Read the model definition and answer for the solid it produces. Units are mm, in the model's axes. A direction names the side the tool comes from. Give positions to 0.01 mm unless a question says otherwise; leave off trailing zeros. Loops run counter-clockwise (first coordinate to the right, second up) from the corner with the lowest first, then second, coordinate; pieces in that order, holes last. Notation, with made-up numbers: (24, 27.5) -> (72, 27.5) arc R24 ccw to (72, 49.5) -> close; hole circle Ø5 at (27, -22.5). An arc over 180 degrees is marked (long way). Write each question's results on one line, items separated by ' | '. Start each with the question number.
Item 1: Section C-C on y = 861 is taken. Write down the section's boundary in (x, z).
Item 2: Section A-A on z = 200 is taken. Write down the section's boundary in (x, y).
Item 3: Which of the six approach directions +Z, -Z, +X, -X, +Y, -Y give full straight-line access (tool end or side, diameter ignored) to faces 1 (the cylindrical face through (323.846, 591.6, -207.509)), 2 (the flat face through (-350, 1323, 3))?
Item 4: Section D-D on x = 202.5 is taken. Write down the section's boundary in (y, z), and give its area (3 significant figures).
Item 5: Determine the mould class of faces 3 (the cylindrical face through (-276.154, 591.6, -207.509)), 4 (the cylindrical face through (323.846, 591.6, 192.491)), 5 (the flat face through (-5, 1323, 250)), 6 (the flat face through (300, 0, -200)) for opening direction Z: +Z half, -Z half, draft (parallel to the pull), parting line (faces both ways), or undercut.
Item 6: Section B-B on x = 300 is taken. Write down the section's boundary in (y, z), and give its area (3 significant figures).
Item 7: Each of these flat-tipped pins is pushed along its axis until it touches: P1, Ø1, axis at x = 280, z = -185.5, coming from the -Y side; P2, Ø6, axis at x = -64.5, z = -10.5, coming from the -Y side; P3, Ø6, axis at y = 575, z = -174, coming from the +X side. Where does it stop, or does it pass through?
Item 8: Find the intervals of material crossed by line 1 (X direction, y = 322.5, z = -197); line 2 (Y direction, x = -314.5, z = 5); line 3 (Z direction, x = -280.5, y = 1076.5), in increasing order.
```python
from build123d import *

# Parameters (mm, degrees)
SKETCH_1_R        = 25
EXTRUDE_1_DEPTH   = 1200
EXTRUDE_1_2_DEPTH = 1200
EXTRUDE_1_3_DEPTH = 1200
EXTRUDE_1_4_DEPTH = 1200
SKETCH_2_W        = 700
SKETCH_2_H        = 500
EXTRUDE_2_DEPTH   = 250


with BuildPart() as part:
    # Sketch 1 → Extrude 1 (new body)
    with BuildSketch(Plane(origin=(0, 0, 0), x_dir=(1, 0, 0), z_dir=(0, 1, 0))):
        with Locations((-300, 200)):
            Circle(SKETCH_1_R)
    extrude(amount=EXTRUDE_1_DEPTH)



with BuildPart() as body_2:
    # Sketch 1 → Extrude 1 2 (new body)
    with BuildSketch(Plane(origin=(0, 0, 0), x_dir=(1, 0, 0), z_dir=(0, 1, 0))):
        with Locations((300, 200)):
            Circle(SKETCH_1_R)
    extrude(amount=EXTRUDE_1_2_DEPTH)


with BuildPart() as body_3:
    # Sketch 1 → Extrude 1 3 (new body)
    with BuildSketch(Plane(origin=(0, 0, 0), x_dir=(1, 0, 0), z_dir=(0, 1, 0))):
        with Locations((300, -200)):
            Circle(SKETCH_1_R)
    extrude(amount=EXTRUDE_1_3_DEPTH)


with BuildPart() as body_4:
    # Sketch 1 → Extrude 1 4 (new body)
    with BuildSketch(Plane(origin=(0, 0, 0), x_dir=(1, 0, 0), z_dir=(0, 1, 0))):
        with Locations((-300, -200)):
            Circle(SKETCH_1_R)
    extrude(amount=EXTRUDE_1_4_DEPTH)


with BuildPart() as part_1:
    add(part.part)

    add(body_2.part)  # Extrude 2 merges body 2

    add(body_3.part)  # Extrude 2 merges body 3

    add(body_4.part)  # Extrude 2 merges body 4
    # Sketch 2 → Extrude 2 (add)
    with BuildSketch(Plane(origin=(0, 1200, 0), x_dir=(1, 0, 0), z_dir=(0, 1, 0))):
        Rectangle(SKETCH_2_W, SKETCH_2_H)
    extrude(amount=EXTRUDE_2_DEPTH)


solid = part_1.part
```
Findings:
1) outline: circle Ø50 at (-300, -200); circle Ø50 at (-300, 200); circle Ø50 at (300, -200); circle Ø50 at (300, 200)
2) outline: (-350, 1200) -> (-325, 1200) -> (-325, 0) -> (-275, 0) -> (-275, 1200) -> (275, 1200) -> (275, 0) -> (325, 0) -> (325, 1200) -> (350, 1200) -> (350, 1450) -> (-350, 1450) -> close
3) face 1: -Y | face 2: +Z, -Z, -X, +Y, -Y
4) outline: (1200, -250) -> (1450, -250) -> (1450, 250) -> (1200, 250) -> close | area: 125,000 mm2
5) face 3: undercut | face 4: undercut | face 5: +Z half | face 6: draft
6) outline: (0, -225) -> (1200, -225) -> (1200, -250) -> (1450, -250) -> (1450, 250) -> (1200, 250) -> (1200, 225) -> (0, 225) -> (0, 175) -> (1200, 175) -> (1200, -175) -> (0, -175) -> close | area: 245,000 mm2
7) P1: y = 0 | P2: y = 1200 | P3: x = 309.8
8) line 1: -324.82 to -275.18, 275.18 to 324.82 | line 2: 1200 to 1450 | line 3: -215.64 to -184.36, 184.36 to 215.64
